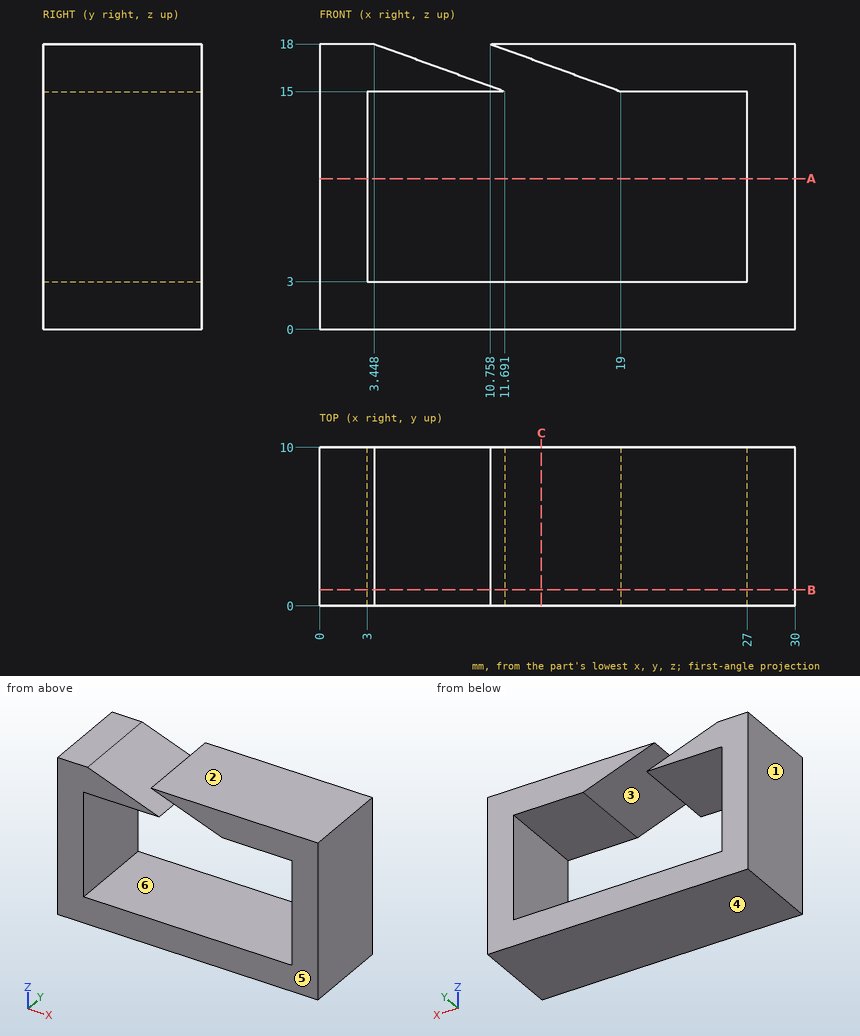
Answer from the drawing. Dimensions are ordinates in mm from the lowest x, y and z of the part. A direction names the side the tool comes from. Coordinates: 2 decimals unless noted, no trailing zeros. Loops run counter-clockwise (first coordinate to the right, second up) from the corner with the lowest first, then second, coordinate; pieces in that order, holes last. Notation, with made-up numbers: (53, 24) -> (79, 24) arc R14 ccw to (79, 33) -> close; hole circle Ø8 at (53, -36). An arc over 180 degrees is marked (long way). Answer as CSV lines item,"result".
Q1. The part is cut by section C-C on x = 14. Write down the section's boundary in (y, z).
Findings:
outline,"(0, 0) -> (10, 0) -> (10, 3) -> (0, 3) -> close; (0, 16.82) -> (10, 16.82) -> (10, 18) -> (0, 18) -> close"
Q2. Find the intervals of material crossed by probe 1 along Z at (x, y) = (22, 0.5); probe 2 along X at (y, z) = (8, 4.5); probe 3 along Z at (x, y) = (11.25, 0.5), in increasing order.
Findings:
probe 1,"z = 0 to 3, 15 to 18"
probe 2,"x = 0 to 3, 27 to 30"
probe 3,"z = 0 to 3, 15 to 15.16, 17.82 to 18"
Q3. The part is cut by section A-A on z = 9.5. Write down the section's boundary in (x, y).
Findings:
outline,"(0, 0) -> (3, 0) -> (3, 10) -> (0, 10) -> close; (27, 0) -> (30, 0) -> (30, 10) -> (27, 10) -> close"
Q4. The part is cut by section B-B on y = 1. Write down the section's boundary in (x, z).
Findings:
outline,"(0, 0) -> (30, 0) -> (30, 18) -> (10.76, 18) -> (19, 15) -> (27, 15) -> (27, 3) -> (3, 3) -> (3, 15) -> (11.69, 15) -> (3.45, 18) -> (0, 18) -> close"
Q5. A tool of negligible diameter and unlimited length cuts with its end or side. For the marked faces 5 and 6, from which of +Z, -Z, +X, -X, +Y, -Y can it reach the whole face along a straight path? Write none if from no direction.
Findings:
face 5,"+Z, -Z, +X, -X, -Y"
face 6,"+Y, -Y"
Q6. For a pull along Z with two mould halves and no side action, classify the marked faces 1, 2, 3 and 4 as +Z half, -Z half, draft (parallel to the pull), parting line (faces both ways), or undercut.
Findings:
face 1,"draft"
face 2,"+Z half"
face 3,"undercut"
face 4,"-Z half"
